Autodesk Inventor part; units mm, degrees
ref_plane "YZ Plane" through (0, 0, 0) normal (1, 0, 0) x (0, 1, 0)
ref_plane "XZ Plane" through (0, 0, 0) normal (0, 1, 0) x (-1, 0, 0)
ref_plane "XY Plane" through (0, 0, 0) normal (0, 0, 1) x (1, 0, 0)
sketch "Sketch1" plane through (0, 0, 0) normal (0, 1, 0) x (-1, 0, 0)
  line L0 (-62.1475, 5) -> (-62.1475, 11)
  line L1 (-62.1475, 11) -> (-2.0643, 11)
  line L2 (-2.0643, 5) -> (-2.0643, 11)
  line L3 (-2.0643, 11) -> (-62.1475, 11)
  line L4 (-2.0643, 5) -> (-62.1475, 5)
  line L5 (-4.3424, 5) -> (-59.9525, 5)
  line L6 (-62.1475, 11) -> (-2.0643, 11)
  line L7 (-43.2275, 5) -> (-43.2275, 11)
  line L8 (-40.0775, 5) -> (-40.0775, 11)
  line L9 (-62.2307, 5) -> (-2.0643, 5)
  line L10 (-32.0775, 5) -> (-32.0775, 11)
  line L11 (-51.2275, 5) -> (-51.2275, 11)
  point P0 (0, 0)
  dimension "d0" = 18.92
  dimension "d1" = 3.15
  dimension "d2" = 8
  dimension "d3" = 8
extrude "Extrusion1" add sketch "Sketch1" along normal blind 20 contours L1 L7 L4 L11 | L1 L10 L4 L8
sketch "Sketch2" plane through (0, 0, 0) normal (0, 1, 0) x (-1, 0, 0)
  line L0 (4.7021, 0) -> (4.7021, 5)
  line L1 (4.7021, 0) -> (4.7021, 11)
  line L2 (-32.0775, 11) -> (4.7021, 11)
  line L3 (4.7021, 11) -> (-32.0775, 11)
  line L4 (-32.0775, 11) -> (-32.0775, 5)
  line L5 (-4.3424, 5) -> (-2.0643, 5)
  line L6 (-32.0775, 5) -> (-2.0643, 5)
  line L7 (-2.0643, 5) -> (-2.0643, 2)
  line L8 (0, 2) -> (-2.0643, 2)
  line L9 (-2.0643, 2) -> (0, 2)
  line L10 (0, 2) -> (0, 0)
  line L11 (4.7021, 0) -> (0, 0)
  line L12 (0, 0) -> (4.7021, 0)
  line L13 (-51.2275, 5) -> (-51.2275, 11)
  line L14 (-51.2275, 5) -> (-51.2275, 11)
  line L15 (-69.0002, 11) -> (-51.2275, 11)
  line L16 (-51.2275, 11) -> (-69.0002, 11)
  line L17 (-69.0002, 0) -> (-69.0002, 5)
  line L18 (-69.0002, 11) -> (-69.0002, 0)
  line L19 (4.7021, 0) -> (0, 0)
  line L20 (-69.0002, 0) -> (-64.295, 0)
  line L21 (-64.295, 0) -> (-64.295, 1.7012)
  line L22 (0, 2) -> (-2.0643, 2)
  line L23 (-2.0643, 2) -> (-2.0643, 5)
  line L24 (-62.2307, 2) -> (-62.2307, 5)
  line L25 (-62.2307, 5) -> (-51.2275, 5)
  line L26 (-64.295, 2) -> (-62.2307, 2)
  line L27 (-64.295, 2) -> (-64.295, 1.7012)
  point P0 (-68.997, 0)
extrude "Extrusion2" add sketch "Sketch2" along normal blind 1
sketch "Sketch3" plane through (40.0775, 0, 11) normal (1, 0, 0) x (0, 0, -1)
  line L0 (6, 1) -> (6, 20)
  line L1 (6, 20) -> (6, 15)
  line L2 (6, 15) -> (0, 15)
  line L3 (0, 1) -> (0, 20)
  line L4 (0, 20) -> (6, 20)
  point P0 (11, 0)
  dimension "d8" = 5
extrude "Extrusion3" add sketch "Sketch3" along normal blind 5.5
sketch "Sketch4" plane through (51.2275, 20, 11) normal (1, 0, 0) x (0, 0, -1)
  line L0 (6, -19) -> (6, 0)
  line L1 (0, -19) -> (0, 0)
  circle A0 centre (3, -16.8) radius 0.9682
  line L2 (0, -19) -> (11, -19)
  point P0 (11, -20)
  dimension "d11" = 6
  dimension "d12" = 3
  dimension "d13" = 2.2
hole "Hole1" at (51.2275, 3.2, 8) direction (-1, 0, 0) diameter 2.4 depth 24 tip angle 118 counterbore diameter 4.6 counterbore depth 1.5
properties part number "screw_supp"
Input: part model. Units: mm. Frame: model coordinates. A direction names the side the tool comes from. Round coordinates to 2 decimals unless told otherwise and drop trailing zeros. Write each loop counter-clockwise with the first axis right and the second up, starting at its lowest first coordinate (ties: lowest second). Pieces come first, ordered by that corner, then holes.
1) Reachability of faces 1 (the flat face through (32.078, 10, 8)), 2 (the flat face through (51.228, 12, 8)), 3 (the flat face through (42, 15, 8)) from +Z, -Z, +X, -X, +Y, -Y: full face, straight path, thin tool, end or side. Return the list, or none.
2) Cut plane D-D (x = 33.5). Return the cut outline in (y, z).
3) Ray query, L1, parallel to X at y = 10, z = 8.5; L2, parallel to Y at x = 50.2, z = 8; L3, parallel to Z at x = 45.5, y = 3.2. Return the intervals inside material, ascending.
4) Cut plane A-A (y = 11.5). Return the cut outline in (x, z).
5) Contact query for flat-ended pins moving along their axis: P1, Ø1.5, axis at x = 7.5, z = 6.5, coming from the +Y side; P2, Ø1.8, axis at y = 7.5, z = 9, coming from the -X side; P3, Ø0.8, axis at x = 63.5, y = 0.5, coming from the -Z side; P4, Ø1.5, axis at x = 55, z = 3, coming from the +Y side. Output: stop coordinate, or through.
6) Cut plane C-C (y = 3.2). Return the cut outline in (x, z).
7) Draft query along Y for faces 4 (the flat face through (43.228, 7, 8)), 5 (the cylindrical face through (36.02, 3.15, 9.2)), 6 (the flat face through (18, 0, 8)). Return one class per face: pulls with the +Y half, pulls with the -Y half, needs draft (parallel to the pull), parting line crosses it, or undercut.
8) Cut plane B-B (z = 4). Return the cut outline in (x, y).
Geometry says:
1. face 1: +Z, -Z, -X, +Y
1. face 2: +Z, -Z, +X, +Y
1. face 3: +Z, -Z, -Y
2. outline: (0, 5) - (20, 5) - (20, 11) - (0, 11) - close; hole circle Ø2.4 at (3.2, 8)
3. L1: x = 32.08 to 40.08, 43.23 to 51.23
3. L2: y = 0 to 0.9, 5.5 to 20
3. L3: z = 5 to 6.8, 9.2 to 11
4. outline: (32.08, 5) - (40.08, 5) - (40.08, 11) - (32.08, 11) - close; (43.23, 5) - (51.23, 5) - (51.23, 11) - (43.23, 11) - close
5. P1: stops at y = 1
5. P2: stops at x = 32.08
5. P3: stops at z = 2
5. P4: passes through
6. outline: (32.08, 5) - (40.08, 5) - (40.08, 6.8) - (32.08, 6.8) - close; (32.08, 9.2) - (40.08, 9.2) - (40.08, 11) - (32.08, 11) - close; (43.23, 5) - (51.23, 5) - (51.23, 5.7) - (49.73, 5.7) - (49.73, 6.8) - (43.23, 6.8) - close; (43.23, 9.2) - (49.73, 9.2) - (49.73, 10.3) - (51.23, 10.3) - (51.23, 11) - (43.23, 11) - close
7. face 4: needs draft
7. face 5: undercut
7. face 6: pulls with the -Y half
8. outline: (-4.7, 0) - (2.06, 0) - (2.06, 1) - (-4.7, 1) - close; (62.23, 0) - (69, 0) - (69, 1) - (62.23, 1) - close
